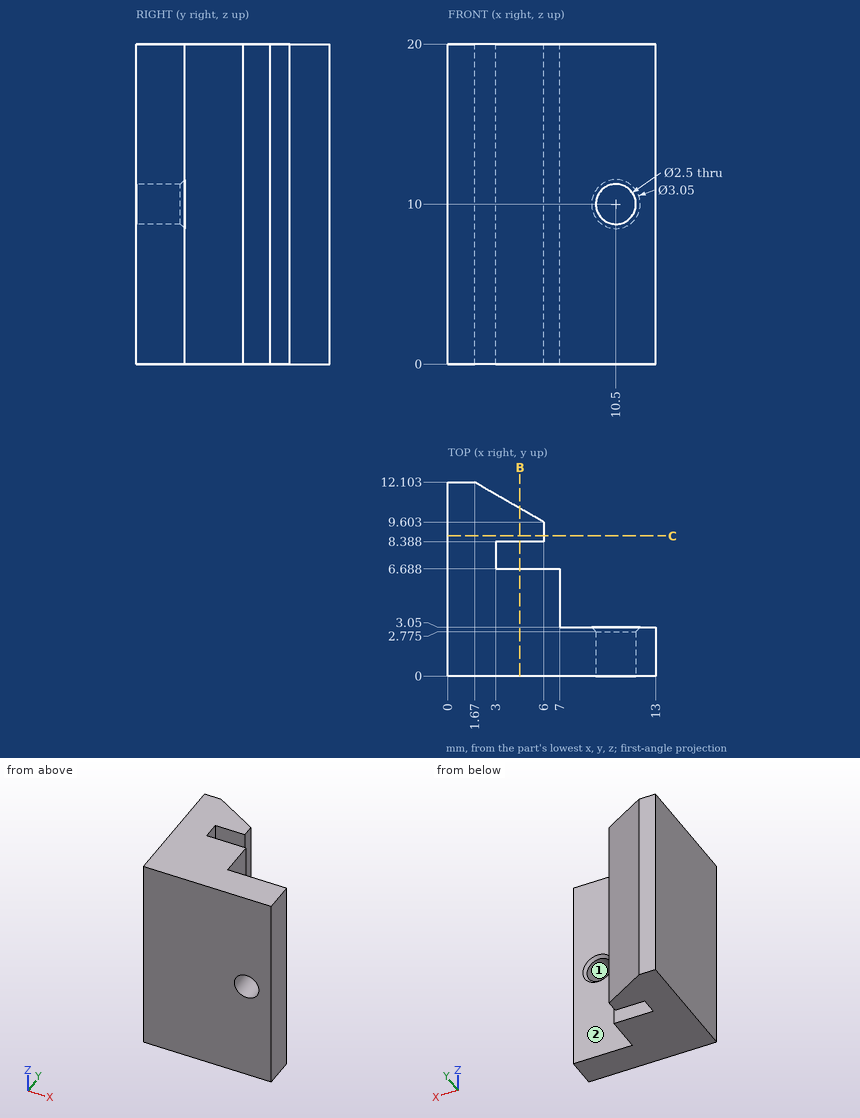
Design review of the part shown in the three views and the two pictorial views. Dimensions are in mm from the part's minimum x, y and z. A direction names the side the tool comes from. Round coordinates to 2 decimals unless told otherwise and drop trailing zeros. Loops run counter-clockwise (first coordinate to the right, second up) from the corner with the lowest first, then second, coordinate; pieces in that order, holes last.
Q1. To check wall thickness, follow line 1 along X through (y, z) = (1.15, 10); line 2 along Z through (x, y) = (10.5, 0.7); line 3 along Y through (x, z) = (6.5, 7). State the ranges of each line that lie inside material, in increasing order.
Result sheet:
line 1: x = 0 to 9.25, 11.75 to 13
line 2: z = 0 to 8.75, 11.25 to 20
line 3: y = 0 to 6.69
Q2. Add section C-C on y = 8.75. Write out the cut boundary in (x, z).
Result sheet:
outline: (0, 0) - (6, 0) - (6, 20) - (0, 20) - close
Q3. Insertion check: pin 1 Ø4.5 at (x, z) = (6, 11) entering from +Y; pin 2 Ø5 at (x, z) = (11, 15) entering from +Y; pin 3 Ø1.8 at (y, z) = (4, 11) entering from +X. Each pin has a flat end and moves straight along its axis. Give the tip position at first contact, or say it passes through.
Result sheet:
pin 1: stops at y = 10.9
pin 2: stops at y = 3.05
pin 3: stops at x = 7
Q4. Add section B-B on x = 4.5. Write out the cut boundary in (y, z).
Result sheet:
outline: (0, 0) - (6.69, 0) - (6.69, 20) - (0, 20) - close; (8.39, 0) - (10.47, 0) - (10.47, 20) - (8.39, 20) - close
Q5. Machinability: for the marked faces 1 and 2, which of the approach directions +Z, -Z, +X, -X, +Y, -Y give a long, thin tool a straight path to every point of the face, cutting with its end or side? Answer none if there is none.
Result sheet:
face 1: +Y, -Y
face 2: +Z, -Z, +X, +Y
